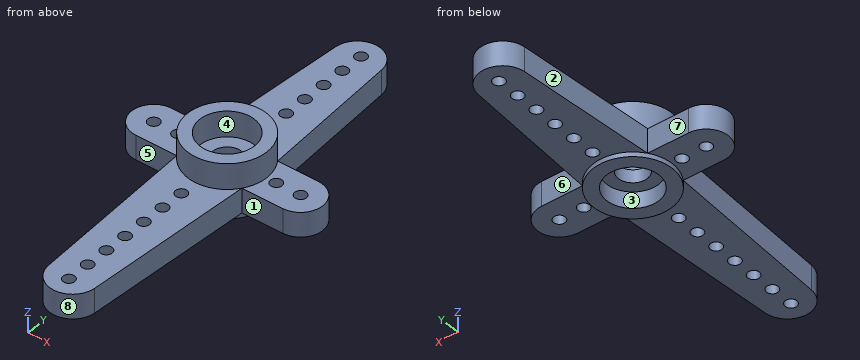
Autodesk Inventor part; units mm, degrees
ref_plane "YZ Plane" through (0, 0, 0) normal (1, 0, 0) x (0, 1, 0)
ref_plane "XZ Plane" through (0, 0, 0) normal (0, 1, 0) x (-1, 0, 0)
ref_plane "XY Plane" through (0, 0, 0) normal (0, 0, 1) x (1, 0, 0)
sketch "스케치1" plane through (0, 0, 0) normal (0, 0, 1) x (1, 0, 0)
  circle A0 centre (0, 0) radius 2.5
  line L0 (-6.35, 0) -> (6.35, 0) construction
  line L1 (-6.35, -1.9) -> (6.35, -1.9)
  line L2 (6.35, 1.9) -> (-6.35, 1.9)
  arc A1 (-6.35, 1.9) -> (-6.35, -1.9) centre (-6.35, 0) ccw
  arc A2 (6.35, -1.9) -> (6.35, 1.9) centre (6.35, 0) ccw
  line L3 (0, 14.5) -> (0, -14.5) construction
  circle A3 centre (0, 14.5) radius 0.5
  circle A4 centre (0, -14.5) radius 0.5
  circle A5 centre (6.35, 0) radius 0.5
  circle A6 centre (-6.35, 0) radius 0.5
  circle A7 centre (-4.25, 0) radius 0.5
  circle A8 centre (4.25, 0) radius 0.5
  line L4 (0, -1.9) -> (0, -18.5)
  line L5 (0, 1.9) -> (0, 15.9)
  arc A9 (1.9954, 14.0355) -> (-1.9954, 14.0355) centre (0, 13.9) ccw
  arc A10 (-1.9969, -16.6117) -> (1.9969, -16.6117) centre (0, -16.5) ccw
  circle A11 centre (0, 0) radius 3.4
  line L6 (-1.9954, 14.0355) -> (-2.8196, 1.9)
  line L7 (1.9954, 14.0355) -> (2.8196, 1.9)
  line L8 (-2.8196, -1.9) -> (-1.9969, -16.6117)
  line L9 (2.8196, -1.9) -> (1.9969, -16.6117)
  circle A12 centre (0, 12.5) radius 0.5
  circle A13 centre (0, 10.5) radius 0.5
  circle A14 centre (0, 8.5) radius 0.5
  circle A15 centre (0, 6.5) radius 0.5
  circle A16 centre (0, 4.5) radius 0.5
  circle A17 centre (0, 0) radius 2.35
  circle A18 centre (0, -16.5) radius 0.5
  circle A19 centre (0, -12.5) radius 0.5
  circle A20 centre (0, -10.5) radius 0.5
  circle A21 centre (0, -8.5) radius 0.5
  circle A22 centre (0, -6.5) radius 0.5
  circle A23 centre (0, -4.5) radius 0.5
  dimension "d0" = 5
  dimension "d1" = 1.9
  dimension "d2" = 16.5
  dimension "d3" = 29
  dimension "d4" = 1
  dimension "d5" = 1
  dimension "d6" = 1
  dimension "d7" = 1
  dimension "d10" = 2.1
  dimension "d17" = 2.1
  dimension "d24" = 16.6
  dimension "d25" = 14
  dimension "d26" = 4
  dimension "d27" = 4
  dimension "d28" = 6.8
  dimension "d31" = 2
  dimension "d36" = 4.7
  dimension "d39" = 2
  dimension "d46" = 2
extrude "돌출1" add sketch "스케치1" along normal blind 2.2 contours A0 L1 A17 L2 | A0 L2 A11 L1 | L2 A17 L5 A0 | A0 L5 A11 L2 | L1 A11 L4 A0 | A0 L4 A17 L1 | L5 A17 L2 A0 | A0 L2 A11 L5 | A17 L1 L2 | L2 L5 A17 | L4 A11 L1 A0 | A0 L1 A17 L4 | A17 L4 L1 | L2 A17 L1 A0 | A0 L1 A11 L2 | L5 L2 A17 | A17 L1 L4
extrude "돌출2" add sketch "스케치1" against normal blind 2.11 contours A0 L1 A17 L2 | A0 L2 A11 L1 | L2 A17 L5 A0 | A0 L5 A11 L2 | L1 A11 L4 A0 | A0 L4 A17 L1 | L5 A17 L2 A0 | A0 L2 A11 L5 | L2 A2 L1 A11 | A11 L5 A16 A15 A14 A13 A12 A3 A9 L7 | A17 L1 L2 | L2 L5 A17 | L4 A11 L1 A0 | A0 L1 A17 L4 | A17 L4 L1 | L9 A10 L4 A18 A4 A19 A20 A21 A22 A23 A11 | L2 A17 L1 A0 | A0 L1 A11 L2 | L5 L2 A17 | A11 L6 A9 L5 A3 A12 A13 A14 A15 A16 | A17 L1 L4 | L4 A23 A22 A21 A20 A19 A4 A18 A10 L8 A11 | A11 L1 A1 L2
extrude "돌출3" cut sketch "스케치1" along normal blind 3.65 contours A17 L1 L2 | L2 L5 A17 | A17 L4 L1 | L5 L2 A17 | A17 L1 L4
sketch "스케치2" plane through (0, 0, 0) normal (0, 0, 1) x (1, 0, 0)
  circle A0 centre (0, 0) radius 1.25
  dimension "d57" = 2.5
extrude "돌출4" cut sketch "스케치2" against normal blind 7.6
sketch "스케치3" plane through (0, 0, -2.11) normal (0, 0, -1) x (-1, 0, 0)
  circle A0 centre (0, 0) radius 2.25
  dimension "d60" = 4.5
extrude "돌출5" cut sketch "스케치3" against normal blind 1
sketch "스케치4" plane through (0, 0, -2.11) normal (0, 0, -1) x (-1, 0, 0)
  point P0 (0, 0)
sketch "스케치5" plane through (0, 0, -2.11) normal (0, 0, -1) x (-1, 0, 0)
  circle A0 centre (0, 0) radius 3.4
  circle A1 centre (0, 0) radius 2.25
  dimension "d63" = 4.5
  dimension "d64" = 6.8
extrude "돌출6" add sketch "스케치5" along normal blind 0.4
sketch "스케치6" plane through (0, 0, -2.11) normal (0, 0, -1) x (-1, 0, 0)
  line L0 (0.9014, 15.3127) -> (-1.0592, 15.3127)
  line L1 (-1.0592, 15.3127) -> (-1.0592, 3.6394)
  line L2 (-1.0592, 3.6394) -> (0.9014, 3.6394)
  line L3 (0.9014, 3.6394) -> (0.9014, 15.3127)
  line L4 (1.0141, -3.7747) -> (-1.0592, -3.7747)
  line L5 (-1.0592, -3.7747) -> (-1.0592, -17.386)
  line L6 (-1.0592, -17.386) -> (1.0141, -17.386)
  line L7 (1.0141, -17.386) -> (1.0141, -3.7747)
  point P0 (0, 0)
extrude "돌출7" add sketch "스케치6" against normal blind 2.11
sketch "스케치7" plane through (0, 0, -2.11) normal (0, 0, -1) x (-1, 0, 0)
  circle A0 centre (0, 14.3) radius 0.5
  arc A1 (1.9954, 14.0355) -> (-1.9954, 14.0355) centre (0, 13.9) ccw
  line L0 (0, 0) -> (0, 0.7105)
  line L1 (0, 0) -> (0.8275, 0)
  circle A2 centre (0, 12.3) radius 0.5
  circle A3 centre (0, 10.3) radius 0.5
  circle A4 centre (0, 8.3) radius 0.5
  circle A5 centre (0, 6.3) radius 0.5
  circle A6 centre (0, 4.3) radius 0.5
  line L2 (0, 15.9) -> (3.4178, 15.9)
  arc A7 (1.9954, 14.0355) -> (-1.9954, 14.0355) centre (0, 13.9) ccw
  circle A8 centre (0, -16.9) radius 0.5
  arc A9 (-1.9969, -16.6117) -> (1.9969, -16.6117) centre (0, -16.5) ccw
  circle A10 centre (0, -14.9) radius 0.5
  circle A11 centre (0, -12.9) radius 0.5
  circle A12 centre (0, -10.9) radius 0.5
  circle A13 centre (0, -8.9) radius 0.5
  circle A14 centre (0, -6.9) radius 0.5
  circle A15 centre (0, -4.9) radius 0.5
  point P0 (0, -18.5)
  dimension "d69" = 1
  dimension "d73" = 2
  dimension "d78" = 1.6
  dimension "d79" = 1
  dimension "d80" = 1.6
  dimension "d86" = 2
extrude "돌출8" cut sketch "스케치7" against normal blind 2.11
sketch "스케치9" plane through (0, 0, -2.11) normal (0, 0, -1) x (-1, 0, 0)
  circle A0 centre (0, 14.3) radius 0.5
  circle A1 centre (0, -16.9) radius 0.5
  point P0 (0, 0)
  dimension "d90" = 14.3
  dimension "d91" = 16.9
properties part number "180도 서보모터 십자축"
Work out the finished part from the listing and answer in its coordinate system (mm). Face numbers are marked on the shaded views. A direction names the side the tool comes from. Give positions to 0.01 mm unless a question says otherwise; leave off trailing zeros. Loops run counter-clockwise (first coordinate to the right, second up) from the corner with the lowest first, then second, coordinate; pieces in that order, holes last. Notation, with made-up numbers: (-9, -27.5) - (0, -27.5) arc R13 cw to (0, -3.5) - close; hole circle Ø11 at (-27.75, -5.5). An arc over 180 degrees is marked (long way). Answer in a Markdown table with one row per item. Add a question column.
Q1. A tool of negligible diameter and unlimited length cuts with its end or side. For the marked faces 4, 5, 6, 7 and 8, from which of +Z, -Z, +X, -X, +Y, -Y can it reach the whole face along a straight path? Write none if from no direction.
Q2. The part is cut by section D-D (z = 1.85). Determine the outline of the cut face in (x, y).
Q3. The part is cut by section A-A (x = -4.25). Determine the outline of the cut face in (y, z), and give its area (3 significant figures).
Q4. Consider line 1 along X through (y, z) = (0, 1); line 2 along X through (y, z) = (-2, 0.1); line 3 along Z through (x, y) = (-2.25, -8). Determine where each line is inside the solid, lowest interval first.
Q5. Determine the mould class of the marked faces 1, 2 and 3 for opening direction X: released by +X, released by -X, zero draft, split by the parting line, or undercut.
Q6. Each of these flat-tipped pins is pushed along its axis until it touches: P1, Ø3, axis at x = -1, y = 9.5, coming from the -Z side; P2, Ø4, axis at x = 0, y = 0, coming from the -Z side; P3, Ø1.7, axis at x = 1, y = 5.5, coming from the +Z side; P4, Ø4, axis at x = 0, y = 1, coming from the +Z side. Where does it stop, or does it pass through?
Q7. The part is cut by section B-B (y = -4.9). Determine the outline of the cut face in (x, z).
Q8. The part is cut by section C-C (z = -0.35). State how many separate pieces and enclosed holes the cut face has, and give its area (3 significant figures).
Solution:
| question | item | result |
|---|---|---|
| 1 | face 4 | +Z |
| 1 | face 5 | +Z, -Z, -X, -Y |
| 1 | face 6 | +Z, -Z, +X, +Y |
| 1 | face 7 | +Z, -Z, -X, +Y |
| 1 | face 8 | +Z, -Z, -Y |
| 2 | outline | circle Ø6.8 at (0, 0); hole circle Ø4.7 at (0, 0) |
| 3 | outline | (-1.9, -2.11) - (-0.5, -2.11) - (-0.5, 0) - (-1.9, 0) - close; (0.5, -2.11) - (1.9, -2.11) - (1.9, 0) - (0.5, 0) - close |
| 3 | area | 5.91 mm² |
| 4 | line 1 | x = -3.4 to -2.35, 2.35 to 3.4 |
| 4 | line 2 | x = -2.75 to -1.23, 1.23 to 2.75 |
| 4 | line 3 | z = -2.11 to 0 |
| 5 | face 1 | zero draft |
| 5 | face 2 | released by -X |
| 5 | face 3 | undercut |
| 6 | P1 | stops at z = -2.11 |
| 6 | P2 | stops at z = -1.11 |
| 6 | P3 | stops at z = 0 |
| 6 | P4 | stops at z = 2.2 |
| 7 | outline | (-2.65, -2.11) - (-0.5, -2.11) - (-0.5, 0) - (-2.65, 0) - close; (0.5, -2.11) - (2.65, -2.11) - (2.65, 0) - (0.5, 0) - close |
| 8 | separate pieces | 1 |
| 8 | enclosed holes | 18 |
| 8 | area | 182 mm² |
